Verification items for the finished model (mm, model axes). Round coordinates to 2 decimals unless told otherwise and drop trailing zeros. Write each loop counter-clockwise with the first axis right and the second up, starting at its lowest first coordinate (ties: lowest second). Pieces come first, ordered by that corner, then holes. Notation, with made-up numbers: (-21, -37) - (-15, -37) arc R12 cw to (-15, -19) - close; hole circle Ø6 at (43.25, 86.5). An arc over 180 degrees is marked (long way). Write each question's results on one line, items separated by ' | '.
```python
from build123d import *

# Parameters (mm, degrees)
F0_R     = 11.1125
F1_DEPTH = 22.225
F2_R     = 2.54
F3_SIZE  = 2.54


with BuildPart() as f1:
    # F0 (on Top) → F1 (new body)
    with BuildSketch(Plane.XY):
        Polygon((10.31875, -17.872599), (20.6375, 0), (10.31875, 17.872599), (-10.31875, 17.872599), (-20.6375, 0), (-10.31875, -17.872599), align=None)
        Circle(F0_R, mode=Mode.SUBTRACT)
    extrude(amount=F1_DEPTH)

    # F2
    f2_edges = [f1.edges().sort_by_distance(p)[0] for p in [
        (0, -17.872599, 22.225),
        (15.478125, -8.9363, 22.225),
        (15.478125, 8.9363, 22.225),
        (0, 17.872599, 22.225),
        (-15.478125, 8.9363, 22.225),
        (-15.478125, -8.9363, 22.225),
        (0, -17.872599, 0),
        (-15.478125, -8.9363, 0),
        (-15.478125, 8.9363, 0),
        (0, 17.872599, 0),
        (15.478125, 8.9363, 0),
        (15.478125, -8.9363, 0),
    ]]
    fillet(f2_edges, radius=F2_R)

    # F3
    f3_edges = [f1.edges().sort_by_distance(p)[0] for p in [
        (-11.1125, 0, 22.225),
    ]]
    chamfer(f3_edges, length=F3_SIZE)


solid = f1.part
```
(1) Section check B-B (z = 15.25). Record the cut outline in (x, y) (1 decimal).
Answer:
outline: (-20.6, 0) - (-10.3, -17.9) - (10.3, -17.9) - (20.6, 0) - (10.3, 17.9) - (-10.3, 17.9) - close; hole circle Ø22.2 at (0, 0)
(2) Section check A-A (x = 0). Record the cut outline in (y, z) (1 decimal), plus the area to 3 significant figures.
Answer:
outline: (-17.9, 2.5) arc R2.5 ccw to (-15.3, 0) - (-11.1, 0) - (-11.1, 19.7) - (-13.7, 22.2) - (-15.3, 22.2) arc R2.5 ccw to (-17.9, 19.7) - close; (11.1, 0) - (15.3, 0) arc R2.5 ccw to (17.9, 2.5) - (17.9, 19.7) arc R2.5 ccw to (15.3, 22.2) - (13.7, 22.2) - (11.1, 19.7) - close | area: 288 mm2
(3) Thickness scan on L1, parallel to Y at x = 0, z = 14.75; L2, parallel to Y at x = 9.5, z = 9.25; L3, parallel to X at y = -6, z = 3.5. Record the ranges inside material, lowest first.
Answer:
L1: -17.87 to -11.11, 11.11 to 17.87 | L2: -17.87 to -5.77, 5.77 to 17.87 | L3: -17.17 to -9.35, 9.35 to 17.17
(4) Mould release check, pull along Y, two halves, no side actions. Record for faces 1 (the flat face through (0, -17.873, 11)), 2 (the cylindrical face through (10.6, 3.34, 9.7)), 3 (the flat face through (12, 0, 0)): released by +Y, released by -Y, zero draft, split by the parting line, or undercut.
Answer:
face 1: released by -Y | face 2: undercut | face 3: zero draft
(5) Go/stop test with flat-tipped pins: pin 1 Ø2 at (y, z) = (2.5, 15.5) entering from -X; pin 2 Ø1 at (x, y) = (-0.5, 13) entering from +Z; pin 3 Ø6 at (y, z) = (-2.5, 18) entering from -X. Record where each tip stops, or that it passes through.
Answer:
pin 1: x = -19.77 | pin 2: z = 22.08 | pin 3: x = -20.64
